Geometry check sheet. Reference: drawing and pictorial views, mm from the part's lowest x, y, z. A direction names the side the tool comes from. Round coordinates to 2 decimals unless told otherwise and drop trailing zeros. Write each loop counter-clockwise with the first axis right and the second up, starting at its lowest first coordinate (ties: lowest second). Pieces come first, ordered by that corner, then holes. Notation, with made-up numbers: M 50.25,6 L 101.25,6 A22 ccw 101.25,41 Z; hole C -28,67 d7. An arc over 180 degrees is marked long. One line per item, written item: value. Start each with the question number.
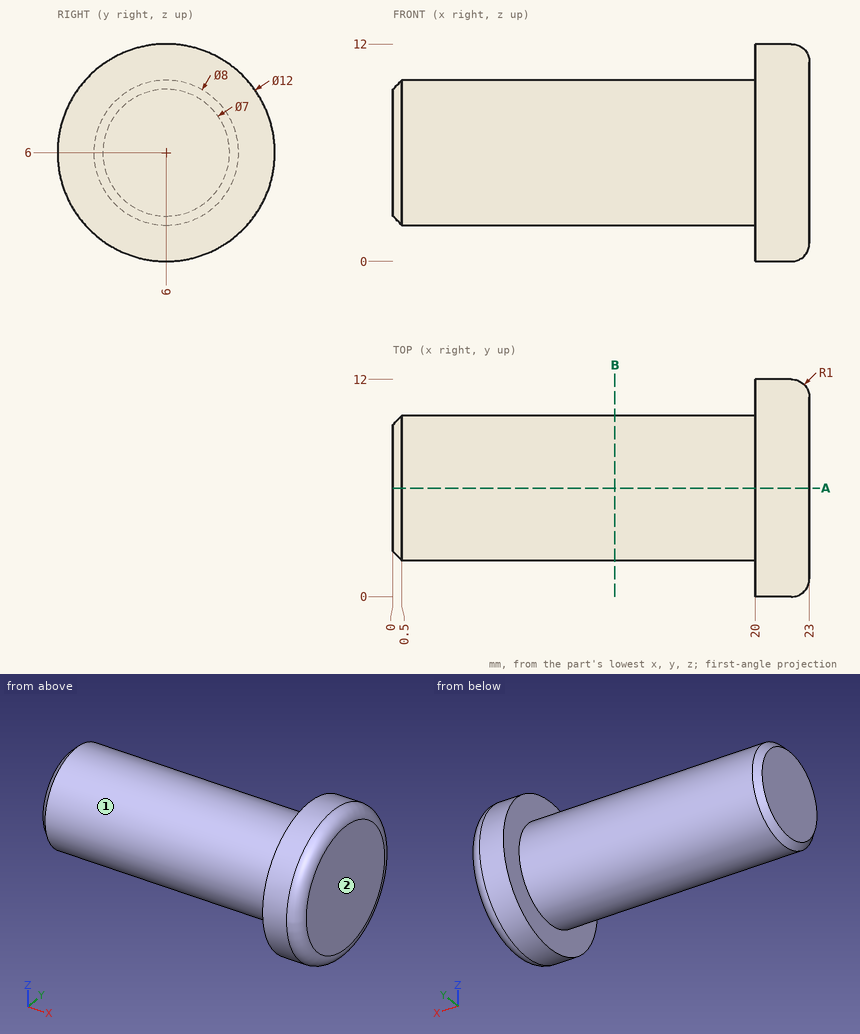
1) Thickness scan on line 1 (X direction, y = 6.75, z = 10); line 2 (Y direction, x = 21, z = 8.25); line 3 (Z direction, x = 4.25, y = 4.25). Record the ranges inside material, lowest first.
2) Access from +Z, -Z, +X, -X, +Y, -Y to the whole of each face (thin tool, end or side, straight path). Record for the marked faces 1 and 2.
3) Cross-section at A-A (y = 6). Record the boundary of the cut face in (x, z), then the cut area to 3 significant figures.
4) Cross-section at B-B (x = 12.25). Record the boundary of the cut face in (y, z).
5) Gauge pin test, flat ends, axial feed: pin 1 Ø1 at (x, z) = (3, 3.5) entering from +Y; pin 2 Ø4 at (x, y) = (12.5, 4.5) entering from -Z; pin 3 Ø6 at (x, y) = (12.5, 3) entering from +Z; pin 4 Ø6 at (y, z) = (4.5, 6.5) entering from -X. Record the tip position at first contact, or that the pin passes through.
Results below:
1. line 1: x = 20 to 23
1. line 2: y = 0.44 to 11.56
1. line 3: z = 2.4 to 9.6
2. face 1: -X
2. face 2: +Z, -Z, +X, +Y, -Y
3. outline: M 0,2.5 L 0.5,2 L 20,2 L 20,0 L 22,0 A1 ccw 23,1 L 23,11 A1 ccw 22,12 L 20,12 L 20,10 L 0.5,10 L 0,9.5 Z
3. area: 195 mm²
4. outline: C 6,6 d8
5. pin 1: stops at y = 9.46
5. pin 2: stops at z = 2
5. pin 3: stops at z = 10
5. pin 4: stops at x = 0
